```python
from build123d import *

# Parameters (mm, degrees)
SKETCH2_R           = 18
BOSS_EXTRUDE1_DEPTH = 5
SKETCH3_R           = 4
CUT_EXTRUDE1_DEPTH  = 122
SKETCH4_R           = 1.5
CUT_EXTRUDE2_DEPTH  = 5


with BuildPart() as part:
    # Sketch2 → Boss-Extrude1 (new body)
    with BuildSketch(Plane.XY):
        Circle(SKETCH2_R)
    extrude(amount=BOSS_EXTRUDE1_DEPTH)

    # Sketch3 → Cut-Extrude1 (cut)
    with BuildSketch(Plane.XY.offset(5)):
        Circle(SKETCH3_R)
    extrude(amount=-CUT_EXTRUDE1_DEPTH, mode=Mode.SUBTRACT)

    # Sketch4 → Cut-Extrude2 (cut)
    with BuildSketch(Plane(origin=(0, 0, 0), x_dir=(-1, 0, 0), z_dir=(0, 0, -1))):
        with Locations((0, 14)):
            Circle(SKETCH4_R)
        with Locations((14, 0)):
            Circle(SKETCH4_R)
        with Locations((0, -14)):
            Circle(SKETCH4_R)
        with Locations((-14, 0)):
            Circle(SKETCH4_R)
    extrude(amount=-CUT_EXTRUDE2_DEPTH, mode=Mode.SUBTRACT)


solid = part.part
```
Geometry: final body of the model. Coordinates: model frame, mm. Round coordinates to 2 decimals unless told otherwise and drop trailing zeros. Order: outer loops, then holes, each group sorted by start corner. A loop starts at its lowest first (then second) coordinate and runs counter-clockwise, first axis right, second up. Notation, with made-up numbers: M -4.75,-14.75 L 2.25,-14.75 A16 cw 2.25,13.25 Z; hole C -22.75,69 d11. An arc over 180 degrees is marked long. One line per item, written item: value.
(1) Line query: probe 1 along Y at (x, z) = (0, 1.7); probe 2 along X at (y, z) = (1, 1.35); probe 3 along X at (y, z) = (-2.5, 1.7). Output: solid intervals per line, ascending. Write a range as [from, to].
Result sheet:
probe 1: [-18, -15.5], [-12.5, -4], [4, 12.5], [15.5, 18]
probe 2: [-17.97, -15.12], [-12.88, -3.87], [3.87, 12.88], [15.12, 17.97]
probe 3: [-17.83, -3.12], [3.12, 17.83]
(2) Cut plane C-C (x = 14.5). Return the cut outline in (y, z).
Result sheet:
outline: M -10.67,0 L -1.41,0 L -1.41,5 L -10.67,5 Z; M 1.41,0 L 10.67,0 L 10.67,5 L 1.41,5 Z
(3) Pull-direction query (Y, two-part tool) for faces 1 (the cylindrical face through (-0.867, -3.905, 2.535)), 2 (the cylindrical face through (-12.5, 0.07, 2.46)), 3 (the flat face through (-4.3, 0.3, 5)), 4 (the cylindrical face through (-2.343, 17.847, 2.465)); classes: pulls with the +Y half, pulls with the -Y half, needs draft (parallel to the pull), parting line crosses it, or undercut.
Result sheet:
face 1: undercut
face 2: undercut
face 3: needs draft
face 4: parting line crosses it
(4) Cut plane B-B (z = 4.4). Return the cut outline in (x, y), and give its area (3 significant figures).
Result sheet:
outline: C 0,0 d36; hole C -14,0 d3; hole C 0,0 d8; hole C 0,-14 d3; hole C 0,14 d3; hole C 14,0 d3
area: 939 mm2
(5) Pin query (flat end, axial travel): P1, Ø7, axis at x = 0, y = 0, coming from the -Z side; P2, Ø2, axis at y = -2.5, z = 4.5, coming from the +X side; P3, Ø1.5, axis at y = 7.5, z = 2, coming from the +X side; P4, Ø1.5, axis at y = -14, z = 2, coming from the +X side. Return the tip coordinate at first contact, or that it passes through.
Result sheet:
P1: through
P2: x = 17.94
P3: x = 16.69
P4: x = 12.18
(6) Cut plane D-D (x = 1). Return the cut outline in (y, z).
Result sheet:
outline: M -17.97,0 L -15.12,0 L -15.12,5 L -17.97,5 Z; M -12.88,0 L -3.87,0 L -3.87,5 L -12.88,5 Z; M 3.87,0 L 12.88,0 L 12.88,5 L 3.87,5 Z; M 15.12,0 L 17.97,0 L 17.97,5 L 15.12,5 Z
(7) Cut plane A-A (y = 14). Return the cut outline in (x, z), and give its area (3 significant figures).
Result sheet:
outline: M -11.31,0 L -1.5,0 L -1.5,5 L -11.31,5 Z; M 1.5,0 L 11.31,0 L 11.31,5 L 1.5,5 Z
area: 98.1 mm2
